Verification items for the finished model (mm, model axes). Round coordinates to 2 decimals unless told otherwise and drop trailing zeros. Write each loop counter-clockwise with the first axis right and the second up, starting at its lowest first coordinate (ties: lowest second). Pieces come first, ordered by that corner, then holes. Notation, with made-up numbers: (41, 17.25) -> (75, 17.25) arc R12 ccw to (75, 30.25) -> close; hole circle Ø9 at (-26.75, 84). An arc over 180 degrees is marked (long way). Use CSV: the item, a comma, the result in double quotes.
```python
from build123d import *

# Parameters (mm, degrees)
F0_R     = 11.25
F1_DEPTH = 7


with BuildPart() as f1:
    # F0 (on Top) → F1 (new body)
    with BuildSketch(Plane.XY):
        with BuildLine():
            ThreePointArc((-911.060802, 406.806157), (-933.68826, 421.752412), (-938.555022, 395.074575))
            ThreePointArc((-938.555022, 395.074575), (-927.521425, 390.557522), (-916.374451, 394.787059))
            ThreePointArc((-916.374451, 394.787059), (-912.448464, 400.235511), (-911.060802, 406.806157))
        make_face()
        with Locations((-927.310802, 406.806157)):
            Circle(F0_R, mode=Mode.SUBTRACT)
        with BuildLine():
            ThreePointArc((-950.082946, 374.286864), (-941.902099, 368.391997), (-938.773615, 358.806157))
            ThreePointArc((-938.773615, 358.806157), (-938.89105, 356.85607), (-939.241657, 354.934168))
            ThreePointArc((-939.241657, 354.934168), (-927.423679, 358.923807), (-915.475009, 355.344548))
            ThreePointArc((-915.475009, 355.344548), (-913.564408, 367.11288), (-904.135728, 374.409728))
            ThreePointArc((-904.135728, 374.409728), (-913.499845, 382.649578), (-916.374451, 394.787059))
            ThreePointArc((-916.374451, 394.787059), (-927.521425, 390.557522), (-938.555022, 395.074575))
            ThreePointArc((-938.555022, 395.074575), (-941.008882, 382.845087), (-950.082946, 374.286864))
        make_face()
        with Locations((-927.310802, 374.806157)):
            Circle(F0_R, mode=Mode.SUBTRACT)
        with BuildLine():
            ThreePointArc((-904.135728, 374.409728), (-913.564408, 367.11288), (-915.475009, 355.344548))
            ThreePointArc((-915.475009, 355.344548), (-897.857167, 342.649671), (-883.347989, 358.806157))
            ThreePointArc((-883.347989, 358.806157), (-889.842881, 371.802325), (-904.135728, 374.409728))
        make_face()
        with Locations((-899.597989, 358.806157)):
            Circle(F0_R, mode=Mode.SUBTRACT)
        with BuildLine():
            ThreePointArc((-939.241657, 354.934168), (-938.89105, 356.85607), (-938.773615, 358.806157))
            ThreePointArc((-938.773615, 358.806157), (-941.902099, 368.391997), (-950.082946, 374.286864))
            ThreePointArc((-950.082946, 374.286864), (-969.200657, 350.864245), (-939.241657, 354.934168))
        make_face()
        with Locations((-955.023615, 358.806157)):
            Circle(F0_R, mode=Mode.SUBTRACT)
    extrude(amount=F1_DEPTH)


solid = f1.part
```
Q1. Material ranges on L1, parallel to Y at x = -917, z = 2; L2, parallel to X at y = 365.5, z = 1.25; L3, parallel to X at y = 367, z = 0.5, recorded low to high.
Filled in:
L1,"356.29 to 370.31, 379.31 to 402.31, 411.31 to 419.37"
L2,"-969.83 to -964.07, -945.98 to -933.63, -920.99 to -908.64, -890.56 to -884.79"
L3,"-969.06 to -962.73, -947.31 to -935.41, -919.21 to -907.31, -891.89 to -885.57"
Q2. Section check C-C (y = 372). Record the cut outline in (x, z).
Filled in:
outline,"(-964.51, 0) -> (-938.21, 0) -> (-938.21, 7) -> (-964.51, 7) -> close; (-916.42, 0) -> (-890.11, 0) -> (-890.11, 7) -> (-916.42, 7) -> close"
Q3. Section check B-B (x = -957). Record the cut outline in (y, z).
Filled in:
outline,"(342.68, 0) -> (347.73, 0) -> (347.73, 7) -> (342.68, 7) -> close; (369.88, 0) -> (374.94, 0) -> (374.94, 7) -> (369.88, 7) -> close"
Q4. Section check D-D (x = -917.5). Record the cut outline in (y, z), plus the area to 3 significant figures.
Filled in:
outline,"(356.56, 0) -> (369.3, 0) -> (369.3, 7) -> (356.56, 7) -> close; (380.31, 0) -> (401.3, 0) -> (401.3, 7) -> (380.31, 7) -> close; (412.31, 0) -> (419.76, 0) -> (419.76, 7) -> (412.31, 7) -> close"
area,"288 mm²"
Q5. Section check A-A (y = 362). Record the cut outline in (x, z), plus the area to 3 significant figures.
Filled in:
outline,"(-970.96, 0) -> (-965.81, 0) -> (-965.81, 7) -> (-970.96, 7) -> close; (-944.24, 0) -> (-910.39, 0) -> (-910.39, 7) -> (-944.24, 7) -> close; (-888.81, 0) -> (-883.66, 0) -> (-883.66, 7) -> (-888.81, 7) -> close"
area,"309 mm²"
Q6. Mould release check, pull along X, two halves, no side actions. Record for faces 1 (the flat face through (-934, 365, 0)), 2 (the cylindrical face through (-889.206, 354.497, 3.451)): released by +X, released by -X, zero draft, split by the parting line, or undercut.
Filled in:
face 1,"zero draft"
face 2,"undercut"
Q7. Go/stop test with flat-tipped pins: P1, Ø1.5, axis at y = 365.5, z = 3, coming from the +X side; P2, Ø5, axis at x = -937.5, y = 381, coming from the -Z side; P3, Ø1.5, axis at y = 353, z = 3, coming from the -X side. Record where each tip stops, or that it passes through.
Filled in:
P1,"x = -884.47"
P2,"z = 0"
P3,"x = -970.47"
